For this review, take the finished solid that the model builds, in its own axes (mm). Face numbers are marked on the shaded views. A direction names the side the tool comes from. Coordinates: 2 decimals unless noted, no trailing zeros. Write each loop counter-clockwise with the first axis right and the second up, starting at its lowest first coordinate (ties: lowest second). Pieces come first, ordered by that corner, then holes. Notation, with made-up numbers: (29.5, -23) -> (68.5, -23) arc R23 ccw to (68.5, -2) -> close; hole circle Ø7 at (50, -0.75). An arc over 180 degrees is marked (long way). Put each result on its own line as item: value. Start each with the question number.
Item 1: Consider section A-A on x = -29. Give the boundary of the cut face in (y, z).
Item 2: Consider section B-B on x = -9.5. Give the boundary of the cut face in (y, z) (3 decimals).
Item 3: For the marked faces 5, 6, 7, 8 and 9, list the 3-axis set-ups (+Z, -Z, +X, -X, +Y, -Y) from which the entire face can be reached by the end or side of a thin tool; tool diameter is ignored.
Item 4: To check wall thickness, follow L1, parallel to Y at x = -36.5, z = 1.75; L2, parallel to Z at x = -39.5, y = 30.4; L3, parallel to X at y = 23, z = 1.25. State the ranges of each line that lie inside material, in increasing order.
Item 5: Consider section C-C on y = 10. Give the boundary of the cut face in (x, z).
Item 6: The part is to be moulded in two halves that separate along X. For the marked faces 1, 2, 3 and 4, say which applies: +X half, -X half, draft (parallel to the pull), parting line (faces both ways), or undercut.
Item 7: Consider section D-D on z = 3. Give the number of separate pieces and of enclosed holes in the cut face, and give its area (3 significant figures).
Item 8: Insertion check: P1, Ø1.8, axis at y = 20.5, z = 2.5, coming from the +X side; P2, Ø10, axis at x = -37.5, y = 17, coming from the +Z side; P3, Ø3, axis at x = -39.5, z = 3, coming from the +Y side (3 decimals); P4, Ø1.8, axis at x = -34.5, z = 3, coming from the -Y side. Each pin has a flat end and moves straight along its axis. Give the tip position at first contact, or say it passes through.
```python
from build123d import *

# Parameters (mm, degrees)
EXTRUDE_1_DEPTH              = 6
EXTRUDE_2_DEPTH              = 6
HOLE_WIZARD_M3_1_D           = 2.5
HOLE_WIZARD_M3_1_CSINK_D     = 3.05
HOLE_WIZARD_M3_1_CSINK_ANGLE = 90
HOLE_WIZARD_M3_2_D           = 2.5
HOLE_WIZARD_M3_2_CSINK_D     = 3.05
HOLE_WIZARD_M3_2_CSINK_ANGLE = 90


with BuildPart() as part:
    # 草图1 → 凸台-拉伸1 (new body)
    with BuildSketch(Plane.XY):
        with BuildLine():
            Line((0, 0), (-46, 0))
            ThreePointArc((-46, 0), (-47.414213562, 0.585786438), (-48, 2))
            Line((-48, 2), (-48, 33))
            ThreePointArc((-48, 33), (-47.414213562, 34.414213562), (-46, 35))
            Line((-46, 35), (0, 35))
            Line((0, 35), (0, 0))
        make_face()
        with BuildLine():
            Line((-30.514833292, 27.446840468), (-24.85843299, 8.825962624))
            ThreePointArc((-24.85843299, 8.825962624), (-25.194545135, 6.885579165), (-26.953467783, 6))
            Line((-26.953467783, 6), (-39.810438922, 6))
            ThreePointArc((-39.810438922, 6), (-41.358692408, 6.641307592), (-42, 8.189561078))
            Line((-42, 8.189561078), (-42, 26.810438922))
            ThreePointArc((-42, 26.810438922), (-41.358692408, 28.358692408), (-39.810438922, 29))
            Line((-39.810438922, 29), (-32.609868086, 29))
            ThreePointArc((-32.609868086, 29), (-31.305886173, 28.569361571), (-30.514833292, 27.446840468))
        make_face(mode=Mode.SUBTRACT)
        with BuildLine():
            Line((-6, 26.810438922), (-6, 8.189561078))
            ThreePointArc((-6, 8.189561078), (-6.641307592, 6.641307592), (-8.189561078, 6))
            Line((-8.189561078, 6), (-15.390131914, 6))
            ThreePointArc((-15.390131914, 6), (-16.694113827, 6.430638429), (-17.485166708, 7.553159532))
            Line((-17.485166708, 7.553159532), (-23.14156701, 26.174037376))
            ThreePointArc((-23.14156701, 26.174037376), (-22.805454865, 28.114420835), (-21.046532217, 29))
            Line((-21.046532217, 29), (-8.189561078, 29))
            ThreePointArc((-8.189561078, 29), (-6.641307592, 28.358692408), (-6, 26.810438922))
        make_face(mode=Mode.SUBTRACT)
    extrude(amount=EXTRUDE_1_DEPTH)

    # 草图3 → 凸台-拉伸2 (add)
    with BuildSketch(Plane.XY.offset(6)):
        with BuildLine():
            Line((5.667856321, 38.482155184), (0.48165081, 35.295911324))
            ThreePointArc((0.48165081, 35.295911324), (-0.021311116, 35.075399086), (-0.565288435, 35))
            Line((-0.565288435, 35), (-3.393768866, 35))
            Line((-3.393768866, 35), (-3.393768866, 0))
            Line((-3.393768866, 0), (-3.026694271, 0))
            ThreePointArc((-3.026694271, 0), (-2.520753033, -0.065052077), (-2.047724325, -0.255976536))
            Line((-2.047724325, -0.255976536), (2.692773727, -2.916952845))
            ThreePointArc((2.692773727, -2.916952845), (7.458012195, -1.578109188), (6.119168538, 3.187129281))
            Line((6.119168538, 3.187129281), (1.021030054, 6.048859331))
            ThreePointArc((1.021030054, 6.048859331), (0.274030723, 6.782422478), (0, 7.792882796))
            Line((0, 7.792882796), (0, 25.665907397))
            ThreePointArc((0, 25.665907397), (0.254451592, 26.642155703), (0.953060755, 27.369996073))
            Line((0.953060755, 27.369996073), (9.332143679, 32.517844816))
            ThreePointArc((9.332143679, 32.517844816), (10.482155184, 37.332143679), (5.667856321, 38.482155184))
        make_face()
    extrude(amount=-EXTRUDE_2_DEPTH)

    # M3 螺纹孔1 (through all)
    with Locations(Plane.XY.offset(6)):
        with Locations((7.5, 35.5), (4.405971132, 0.135088218)):
            CounterSinkHole(HOLE_WIZARD_M3_1_D / 2, HOLE_WIZARD_M3_1_CSINK_D / 2, counter_sink_angle=HOLE_WIZARD_M3_1_CSINK_ANGLE)

    # M3 螺纹孔2 (through all)
    with Locations(Plane(origin=(0, 35, 0), x_dir=(1, 0, 0), z_dir=(0, 1, 0))):
        with Locations((-39.5, -3), (-9.5, -3)):
            CounterSinkHole(HOLE_WIZARD_M3_2_D / 2, HOLE_WIZARD_M3_2_CSINK_D / 2, counter_sink_angle=HOLE_WIZARD_M3_2_CSINK_ANGLE)


solid = part.part
```
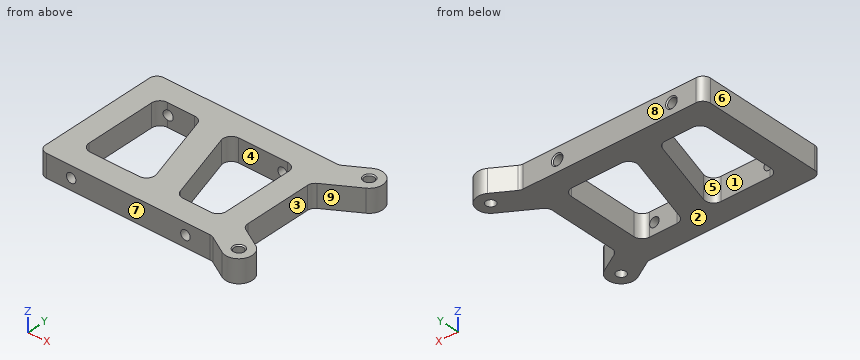
Return value:
1. outline: (0, 0) -> (6, 0) -> (6, 6) -> (0, 6) -> close; (22.46, 0) -> (35, 0) -> (35, 6) -> (22.46, 6) -> close
2. outline: (0, 0) -> (6, 0) -> (6, 1.75) -> (0, 1.75) -> close; (0, 4.25) -> (6, 4.25) -> (6, 6) -> (0, 6) -> close; (29, 0) -> (35, 0) -> (35, 1.475) -> (34.725, 1.75) -> (29, 1.75) -> close; (29, 4.25) -> (34.725, 4.25) -> (35, 4.525) -> (35, 6) -> (29, 6) -> close
3. face 5: +Z, -Z
3. face 6: +Z, -Z, -X, +Y, -Y
3. face 7: +Z, -Z, -X, -Y
3. face 8: +Z, -Z, -X, +Y
3. face 9: +Z, -Z, +X
4. L1: 0 to 6, 29 to 35
4. L2: 0 to 1.75, 4.25 to 6
4. L3: -48 to -42, -29.16 to -22.18, -6 to 0
5. outline: (-48, 0) -> (-42, 0) -> (-42, 6) -> (-48, 6) -> close; (-25.22, 0) -> (-18.23, 0) -> (-18.23, 6) -> (-25.22, 6) -> close; (-6, 0) -> (0, 0) -> (0, 6) -> (-6, 6) -> close
6. face 1: undercut
6. face 2: draft
6. face 3: +X half
6. face 4: undercut
7. separate pieces: 3
7. enclosed holes: 2
7. area: 1,090 mm^2
8. P1: x = 0
8. P2: z = 6
8. P3: y = 34.975
8. P4: y = 0
